Part model, mm, in its own coordinate system. Face numbers are marked on the shaded views. Give positions to 0.01 mm unless a question says otherwise; leave off trailing zeros. Order: outer loops, then holes, each group sorted by start corner. A loop starts at its lowest first (then second) coordinate and runs counter-clockwise, first axis right, second up. Notation, with made-up numbers: M 8,-26 L 18,-26 A8 cw 18,-21 Z; hole C -24,-4.75 d5. An arc over 180 degrees is marked long. Answer as a JSON object with one key per item and string values.
from build123d import *

# Parameters (mm, degrees)
F1_DEPTH = 10
F2_W     = 8.3
F2_H     = 6.3
F3_DEPTH = 3


with BuildPart() as f1:
    # F0 (on Front) → F1 (new body)
    with BuildSketch(Plane.XZ):
        Polygon((14.091946, 0), (0, 0), (34.529055, -44.594892), (34.529055, -15.794892), (26.692673, -5.674065), (26.692673, -16.274065), align=None)
    extrude(amount=F1_DEPTH)

    # F2 (on Top) → F3 (cut)
    with BuildSketch(Plane.XY):
        with Locations((7.079836, -5.139073)):
            Rectangle(F2_W, F2_H)
    extrude(amount=-F3_DEPTH, mode=Mode.SUBTRACT)


solid = f1.part
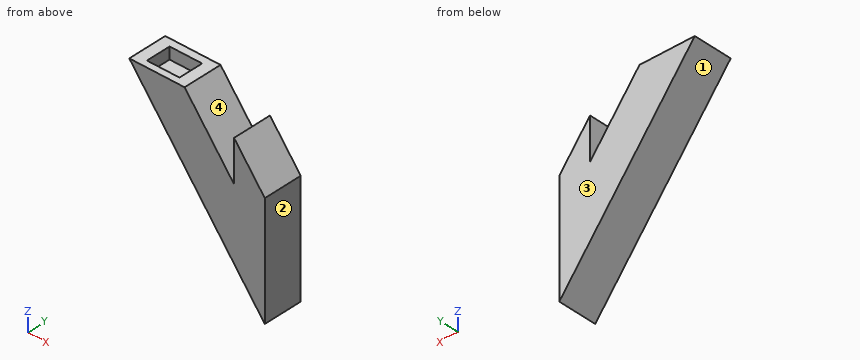
1. Cut at D-D on z = -14. Give the cut face in (x, y), plus the area to 3 significant figures.
Worked answers:
{"outline": "M 10.84,-10 L 24.93,-10 L 24.93,0 L 10.84,0 Z; M 26.69,-10 L 33.14,-10 L 33.14,0 L 26.69,0 Z", "area": "205 mm^2"}
2. Two-plate mould, pull along X, no slides. Class the marked faces 1, 2, 3 and 4: +X half, -X half, draft (parallel to the pull), parting line (faces both ways), or undercut.
Worked answers:
{"face 1": "-X half", "face 2": "+X half", "face 3": "draft", "face 4": "undercut"}
3. Cut at B-B on y = -3. Give the cut face in (x, z), plus the area to 3 significant figures.
Worked answers:
{"outline": "M 0,0 L 34.53,-44.59 L 34.53,-15.79 L 26.69,-5.67 L 26.69,-16.27 L 14.09,0 L 11.23,0 L 11.23,-3 L 2.93,-3 L 2.93,0 Z", "area": "558 mm^2"}
4. Probe line 1 along X through (y, z) = (-7.5, -4.5); line 2 along Z through (x, y) = (17.5, -8); line 3 along Z through (x, y) = (30, -6.25). List the from-to ranges inside material, lowest first.
Worked answers:
{"line 1": "x = 3.48 to 17.58", "line 2": "z = -22.6 to -4.4", "line 3": "z = -38.75 to -9.95"}
5. Cut at C-C on x = 8. Give the cut face in (y, z), plus the area to 3 significant figures.
Worked answers:
{"outline": "M -10,-10.33 L 0,-10.33 L 0,0 L -1.99,0 L -1.99,-3 L -8.29,-3 L -8.29,0 L -10,0 Z", "area": "84.4 mm^2"}
6. Pin check, flat tips, straight feed: P1, Ø1.5, axis at y = -6.5, z = -1.5, coming from the -X side; P2, Ø3, axis at x = 16, y = -2, coming from the -Z side; P3, Ø1.9, axis at x = 8, y = -6.5, coming from the +Z side. Stop position of each tip, or through.
Worked answers:
{"P1": "stops at x = 0.58", "P2": "stops at z = -22.6", "P3": "stops at z = -3"}
7. Cut at A-A on z = -6.5. Give the cut face in (x, y), plus the area to 3 significant figures.
Worked answers:
{"outline": "M 5.03,-10 L 19.12,-10 L 19.12,0 L 5.03,0 Z; M 26.69,-10 L 27.33,-10 L 27.33,0 L 26.69,0 Z", "area": "147 mm^2"}
